Autodesk Inventor part; units mm, degrees
ref_plane "YZ Plane" through (0, 0, 0) normal (1, 0, 0) x (0, 1, 0)
ref_plane "XZ Plane" through (0, 0, 0) normal (0, 1, 0) x (-1, 0, 0)
ref_plane "XY Plane" through (0, 0, 0) normal (0, 0, 1) x (1, 0, 0)
sketch "Sketch1" plane through (0, 0, 0) normal (0, 0, 1) x (1, 0, 0)
  line L0 (0, 0) -> (-68, 0)
  arc A0 (-58.4163, 20.5251) -> (-68, 0) centre (-68, 12.5) ccw
  line L1 (-58.4163, 20.5251) -> (-47.3335, 7.2899)
  arc A1 (-47.3335, 7.2899) -> (-40.2899, 6.6665) centre (-43.5, 10.5) ccw
  line L2 (-40.2899, 6.6665) -> (-34.9101, 11.1715)
  arc A2 (-29.5895, 11.8708) -> (-34.9101, 11.1715) centre (-31.7, 7.338) ccw
  line L3 (-29.5895, 11.8708) -> (-16.9105, 5.9673)
  arc A3 (-16.9105, 5.9673) -> (-13.0552, 5.8143) centre (-14.8, 10.5) ccw
  line L4 (-13.0552, 5.8143) -> (-4.5, 9)
  dimension "d0" = 68
  dimension "d1" = 12.5
  dimension "d2" = 24.5
  dimension "d3" = 36.3
  dimension "d4" = 53.2
  dimension "d5" = 5
  dimension "d6" = 10.5
  dimension "d8" = 9
  dimension "d9" = 63.5
sketch "Sketch2" plane through (0, 0, 0) normal (1, 0, 0) x (0, 1, 0)
  circle A0 centre (0, 0) radius 2
  dimension "d7" = 4
sweep "Sweep1" add profiles "Sketch2" path "Sketch1"
properties part number "B1"
Verification items for the finished model (mm, model axes). Coordinates: 2 decimals unless noted, no trailing zeros. Write item = value, one per line.
Q1. Mould release check, pull along Y, two halves, no side actions. Record for faces 1 (the face through (0, 0, 0)), 2 (the face through (-4.5, 9, 0)), 3 (the face through (-34, 0, 2)): released by +Y, released by -Y, zero draft, split by the parting line, or undercut.
Answer:
face_1 = zero draft
face_2 = released by +Y
face_3 = undercut
Q2. Material ranges on L1, parallel to Y at x = -77.5, z = 1.55; L2, parallel to Y at x = -57, z = 1.5; L3, parallel to X at y = 14, z = 1.65, recorded low to high. Write a range as from..to.
Answer:
L1 = 2.54..6.5, 18.5..22.46
L2 = -1.32..1.32, 16.77..20.89
L3 = -81.55..-79.27, -54.43..-51.48
Q3. Go/stop test with flat-tipped pins: pin 1 Ø6 at (x, y) = (-65.5, 4) entering from +Z; pin 2 Ø10 at (x, y) = (-33, 16.5) entering from -Z; pin 3 Ø1.5 at (y, z) = (2.5, 1) entering from -X; pin 4 Ø1 at (y, z) = (3, -1) entering from -X. Record where each tip stops, or that it passes through.
Answer:
pin_1 = 1.73
pin_2 = -2
pin_3 = -78.95
pin_4 = -79.13
